Source: three-view drawing plus pictorial views. Frame: mm from the lowest corner of the part. Give positions to 0.01 mm unless a question says otherwise; leave off trailing zeros. Write each loop counter-clockwise with the first axis right and the second up, starting at its lowest first coordinate (ties: lowest second). Pieces come first, ordered by that corner, then holes.
Q1. Line query: L1, parallel to Y at x = 50, z = 11.25; L2, parallel to Y at x = 15, z = 1.5; L3, parallel to X at y = 35, z = 7.5. Output: solid intervals per line, ascending.
Q2. Cut plane C-C on z = 5.5. Return the cut outline in (x, y), plus the area to 3 significant figures.
Q3. Pin query (flat end, axial travel): pin 1 (3 mm diameter, centred on x = 115.5, z = 1.5, fed in from -Y); pin 2 (3 mm diameter, centred on y = 31, z = 6.5, fed in from +X); pin 3 (1.5 mm diameter, centred on x = 73, z = 1.5, fed in from -Y). Return the tip coordinate at first contact, or that it passes through.
Q4. Cut plane A-A on y = 77. Return the cut outline in (x, z).
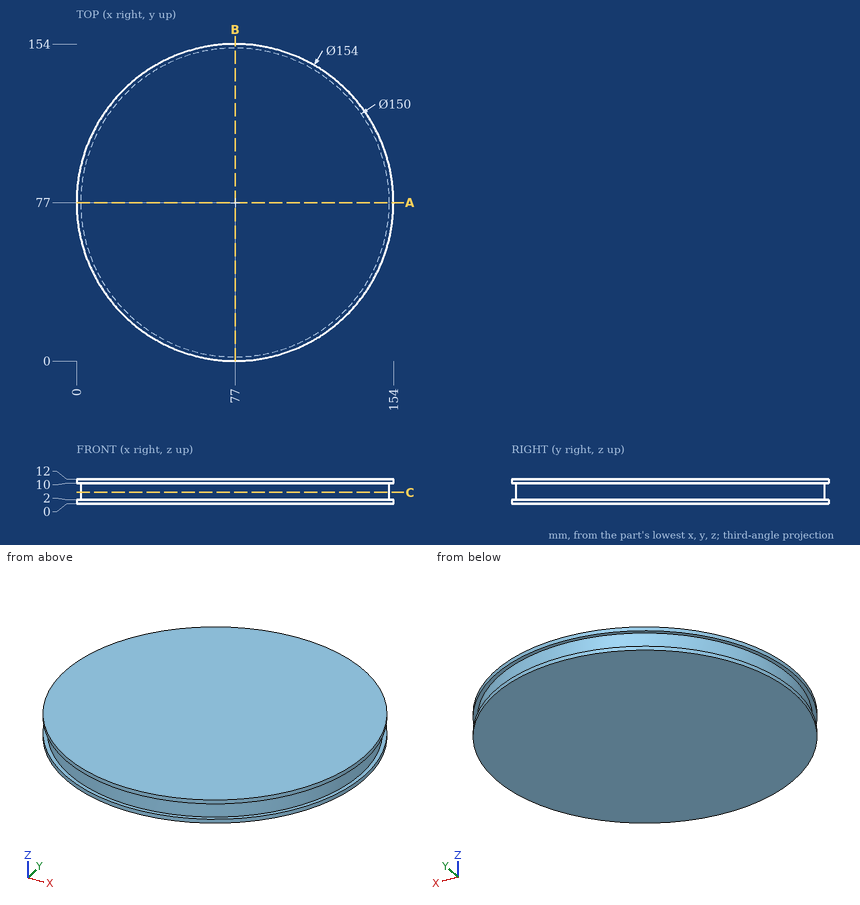
Data:
1. L1: y = 4.89 to 149.11
1. L2: y = 31.34 to 122.66
1. L3: x = 14.86 to 139.14
2. outline: circle Ø150 at (77, 77)
2. area: 17,700 mm2
3. pin 1: stops at y = 9.47
3. pin 2: stops at x = 137.37
3. pin 3: stops at y = 0.07
4. outline: (0, 0) - (154, 0) - (154, 2) - (152, 2) - (152, 10) - (154, 10) - (154, 12) - (0, 12) - (0, 10) - (2, 10) - (2, 2) - (0, 2) - close
